The model under review builds one solid part; all positions refer to its coordinate system, in mm. Face numbers are marked on the shaded views. A direction names the side the tool comes from. Round coordinates to 2 decimals unless told otherwise and drop trailing zeros. Loops run counter-clockwise (first coordinate to the right, second up) from the corner with the lowest first, then second, coordinate; pieces in that order, holes last. Notation, with made-up numbers: M 6,35 L 34,35 A20 ccw 34,47 Z; hole C -40,-3 d8. An arc over 180 degrees is marked long. One line per question, with ' | ' between items.
from build123d import *

# Parameters (mm, degrees)
SKETCH2_W           = 50
SKETCH2_H           = 50
BOSS_EXTRUDE1_DEPTH = 8
BOSS_EXTRUDE2_START = -8
BOSS_EXTRUDE2_DEPTH = 8
CUT_EXTRUDE2_DEPTH  = 8
BOSS_EXTRUDE3_START = -28
BOSS_EXTRUDE3_DEPTH = 6
CUT_EXTRUDE3_DEPTH  = 100.419585885
FILLET1_R           = 3


with BuildPart() as part:
    # Sketch2 → Boss-Extrude1 (new body)
    with BuildSketch(Plane(origin=(0, 0, 0), x_dir=(1, 0, 0), z_dir=(0, 1, 0))):
        Rectangle(SKETCH2_W, SKETCH2_H)
    extrude(amount=BOSS_EXTRUDE1_DEPTH)

    # Sketch5 → Boss-Extrude2 (add)
    with BuildSketch(Plane(origin=(0, 0, -25), x_dir=(-1, 0, 0), z_dir=(0, 0, -1)).offset(BOSS_EXTRUDE2_START)):
        Polygon((-25, 0), (-25, 71.819564568), (25, 90.018076282), (25, 0), align=None)
    extrude(amount=-BOSS_EXTRUDE2_DEPTH)

    # Sketch6 → Cut-Extrude2 (cut)
    with BuildSketch(Plane(origin=(0, 8, 0), x_dir=(1, 0, 0), z_dir=(0, 1, 0))):
        with BuildLine():
            Line((-12.25, 2), (-12.25, -18))
            ThreePointArc((-12.25, -18), (-16.5, -22.25), (-20.75, -18))
            Line((-20.75, -18), (-20.75, 2))
            ThreePointArc((-20.75, 2), (-16.5, 6.25), (-12.25, 2))
        make_face()
        with BuildLine():
            Line((12.25, 2), (12.25, -18))
            ThreePointArc((12.25, -18), (16.5, -22.25), (20.75, -18))
            Line((20.75, -18), (20.75, 2))
            ThreePointArc((20.75, 2), (16.5, 6.25), (12.25, 2))
        make_face()
    extrude(amount=-CUT_EXTRUDE2_DEPTH, mode=Mode.SUBTRACT)

    # Sketch7 → Boss-Extrude3 (add)
    with BuildSketch(Plane(origin=(25, 0, 0), x_dir=(0, 0, -1), z_dir=(1, 0, 0)).offset(BOSS_EXTRUDE3_START)):
        Polygon((9, 8), (-10.543361274, 8), (9, 43.271779749), align=None)
    extrude(amount=BOSS_EXTRUDE3_DEPTH)

    # Sketch8 → Cut-Extrude3 (cut, through all)
    with BuildSketch(Plane.XY.offset(-9)):
        with BuildLine():
            Line((-12.5, 75.401351615), (-12.5, 20.566768933))
            ThreePointArc((-12.5, 20.566768933), (-15.75, 17.316768933), (-19, 20.566768933))
            Line((-19, 20.566768933), (-19, 75.401351615))
            ThreePointArc((-19, 75.401351615), (-15.75, 78.651351615), (-12.5, 75.401351615))
        make_face()
        with BuildLine():
            Line((19, 63.936289235), (19, 20.566768933))
            ThreePointArc((19, 20.566768933), (15.75, 17.316768933), (12.5, 20.566768933))
            Line((12.5, 20.566768933), (12.5, 63.936289235))
            ThreePointArc((12.5, 63.936289235), (15.75, 67.186289235), (19, 63.936289235))
        make_face()
    extrude(amount=-CUT_EXTRUDE3_DEPTH, mode=Mode.SUBTRACT)

    # Fillet1
    fillet1_edges = [part.edges().sort_by_distance(p)[0] for p in [
        (-25, 90.018076282, -13),
        (25, 71.819564568, -13),
        (-25, 4, -25),
        (25, 4, -25),
        (25, 4, 25),
        (-25, 4, 25),
    ]]
    fillet(fillet1_edges, radius=FILLET1_R)


solid = part.part
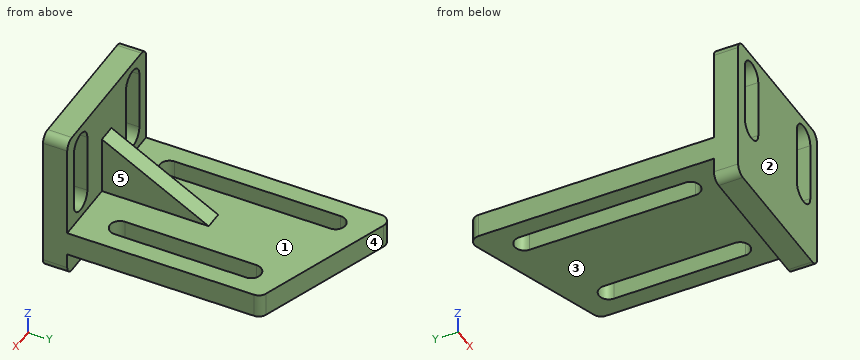
1) Add section A-A on y = 58.5. State the section outline as (x, z) points.
Output values:
outline: M -25,-17 L -19,-17 L -19,-9 L -25,-9 Z; M -12.5,-17 L 12.5,-17 L 12.5,-9 L -12.5,-9 Z; M 19,-17 L 25,-17 L 25,-9 L 19,-9 Z
2) Add section C-C on z = 2. State the section outline as (x, y) points.
Output values:
outline: M -25,0 L -20.75,0 L -20.75,8 L -25,8 Z; M -12.25,0 L 12.25,0 L 12.25,8 L 3,8 L 3,23.42 L -3,23.42 L -3,8 L -12.25,8 Z; M 20.75,0 L 25,0 L 25,8 L 20.75,8 Z
3) Add section B-B on x = 16.5. State the section outline as (y, z) points, then the cut area to 3 significant figures.
Output values:
outline: M 0,-25 L 8,-25 L 8,-17 L 17.4,-17 L 17.4,-9 L 8,-9 L 8,-6.25 L 0,-6.25 Z; M 0,22.25 L 8,22.25 L 8,25 L 0,25 Z; M 67.1,-17 L 74.91,-17 L 74.91,-9 L 67.1,-9 Z | area: 310 mm²
4) Add section D-D on x = -8. State the section outline as (y, z) points, then the cut area to 3 significant figures.
Output values:
outline: M 0,-25 L 8,-25 L 8,-17 L 83.83,-17 L 83.83,-9 L 8,-9 L 8,25 L 0,25 Z | area: 1,010 mm²
5) Machinability: for the marked faces 1, 2, 3, 4 and 5, which of the approach directions +Z, -Z, +X, -X, +Y, -Y give a long, thin tool a straight path to every point of the face, cutting with its end or side? Answer none if there is none.
Output values:
face 1: +Z, +Y | face 2: +Z, -Z, +X, -X, -Y | face 3: -Z, +X, -X, +Y | face 4: +Z, -Z, +X, +Y | face 5: +Z, +X, +Y
6) For line 1 (Y direction, x = 5, z = -7); line 2 (X direction, y = 64.5, z = -15); line 3 (Z direction, x = -11.5, y = 72), list the stretches that pass through material, from the lowest coordinate up.
Output values:
line 1: y = 0 to 8 | line 2: x = -25 to -19, -12.5 to 12.55, 18.95 to 25 | line 3: z = -17 to -9
7) Insertion check: P1, Ø5, axis at x = -13.5, y = 58.5, coming from the -Z side; P2, Ø12, axis at y = 78, z = 2, coming from the +X side; P3, Ø15.5, axis at y = 28.5, z = -4, coming from the -X side; P4, Ø6.5, axis at x = -12, z = -19.5, coming from the +Y side. Each pin has a flat end and moves straight along its axis. Give the tip position at first contact, or say it passes through.
Output values:
P1: stops at z = -17 | P2: passes through | P3: stops at x = -25 | P4: stops at y = 86.04
